Geometry: final body of the model. Coordinates: model frame, mm. A direction names the side the tool comes from. Round coordinates to 2 decimals unless told otherwise and drop trailing zeros. Loops run counter-clockwise (first coordinate to the right, second up) from the corner with the lowest first, then second, coordinate; pieces in that order, holes last. Notation, with made-up numbers: (52, 28.25) - (95, 28.25) arc R31 cw to (95, 61.25) - close; hole circle Ø7 at (84.25, 12). An arc over 180 degrees is marked (long way). Answer as CSV lines item,"result".
from build123d import *

# Parameters (mm, degrees)
SKETCH_1_R      = 10
EXTRUDE_1_DEPTH = 5


with BuildPart() as part:
    # 草图1 → 凸台-拉伸1 (new body)
    with BuildSketch(Plane.XY):
        with BuildLine():
            Line((13, -5), (10, -5))
            Line((10, -5), (10, -8))
            Line((10, -8), (8.94427191, -8))
            ThreePointArc((8.94427191, -8), (0, -12), (-8.94427191, -8))
            Line((-8.94427191, -8), (-10, -8))
            Line((-10, -8), (-10, -5))
            Line((-10, -5), (-13, -5))
            Line((-13, -5), (-13, 5))
            Line((-13, 5), (-10, 5))
            Line((-10, 5), (-10, 8))
            Line((-10, 8), (-8.94427191, 8))
            ThreePointArc((-8.94427191, 8), (0, 12), (8.94427191, 8))
            Line((8.94427191, 8), (10, 8))
            Line((10, 8), (10, 5))
            Line((10, 5), (13, 5))
            Line((13, 5), (13, -5))
        make_face()
        Circle(SKETCH_1_R, mode=Mode.SUBTRACT)
    extrude(amount=EXTRUDE_1_DEPTH)


solid = part.part
(1) Section C-C (z = 3.95). Output: boundary loops of the cut face in (x, y), and give its area (3 significant figures).
Findings below:
outline,"(-13, -5) - (-10, -5) - (-10, -8) - (-8.94, -8) arc R12 ccw to (8.94, -8) - (10, -8) - (10, -5) - (13, -5) - (13, 5) - (10, 5) - (10, 8) - (8.94, 8) arc R12 ccw to (-8.94, 8) - (-10, 8) - (-10, 5) - (-13, 5) - close; hole circle Ø20 at (0, 0)"
area,"165 mm2"
(2) Access query for faces 5 (the face through (-10, 6, 2)), 6 (the face through (11, 5, 2)), 7 (the face through (9.5, -8, 2.5)), 8 (the face through (-10, -7, 2)), 9 (the face through (10, 3, 0)). Directions: +Z, -Z, +X, -X, +Y, -Y. A direction counts if a zero-diameter tool reaches every point of the face in a straight line with its end or side. Return the directions, or none.
Findings below:
face 5,"+Z, -Z, -X, +Y"
face 6,"+Z, -Z, +X, +Y"
face 7,"+Z, -Z, +X, -Y"
face 8,"+Z, -Z, -X, -Y"
face 9,"-Z, +X, -X, +Y, -Y"
(3) Section B-B (y = 0). Output: boundary loops of the cut face in (x, z).
Findings below:
outline,"(-13, 0) - (-10, 0) - (-10, 5) - (-13, 5) - close; (10, 0) - (13, 0) - (13, 5) - (10, 5) - close"
(4) Draft query along Y for faces 1 (the face through (10, 7, 2)), 2 (the face through (-9.5, 8, 2.5)), 3 (the face through (-2.17, -9.76, 2.46)), 4 (the face through (0, -12, 2)). Return one class per face: pulls with the +Y half, pulls with the -Y half, needs draft (parallel to the pull), parting line crosses it, or undercut.
Findings below:
face 1,"needs draft"
face 2,"pulls with the +Y half"
face 3,"undercut"
face 4,"pulls with the -Y half"
(5) Pin query (flat end, axial travel): P1, Ø1.5, axis at x = -11.5, z = 3, coming from the -Y side; P2, Ø1.2, axis at x = 9.5, z = 3, coming from the +Y side; P3, Ø0.9, axis at x = -11, z = 2.5, coming from the +Y side. Return the tip coordinate at first contact, or that it passes through.
Findings below:
P1,"y = -5"
P2,"y = 8.05"
P3,"y = 5"
(6) Section A-A (x = 0). Output: boundary loops of the cut face in (y, z).
Findings below:
outline,"(-12, 0) - (-10, 0) - (-10, 5) - (-12, 5) - close; (10, 0) - (12, 0) - (12, 5) - (10, 5) - close"
(7) Material intervals for line 1 along Y through (x, z) = (0, 1.3); line 2 along X through (y, z) = (6, 2.05); line 3 along Y through (x, z) = (6, 3.45), sorted ascending.
Findings below:
line 1,"-12 to -10, 10 to 12"
line 2,"-10 to -8, 8 to 10"
line 3,"-10.39 to -8, 8 to 10.39"
(8) Section D-D (x = -10.75). Output: boundary loops of the cut face in (y, z), and give its area (3 significant figures).
Findings below:
outline,"(-5, 0) - (5, 0) - (5, 5) - (-5, 5) - close"
area,"50.0 mm2"
